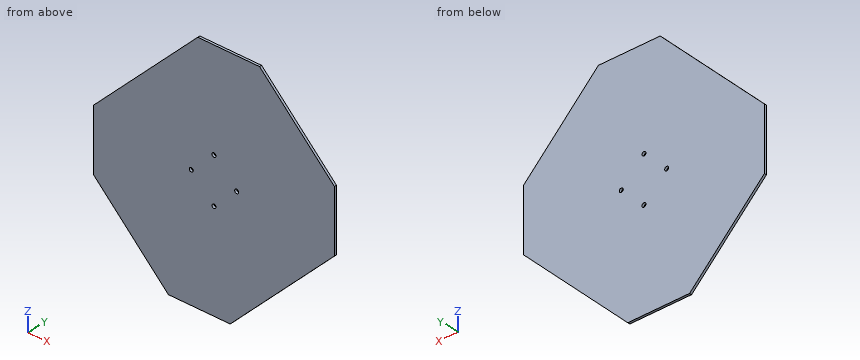
```python
from build123d import *

# Parameters (mm, degrees)
BOSS_EXTRUDE2_DEPTH              = 3
F_13_64_0_20313_DIAMETER_HOLE1_D = 5.159502


with BuildPart() as part:
    # Sketch3 → Boss-Extrude2 (new body)
    with BuildSketch(Plane(origin=(0, 0, 0), x_dir=(1, 0, 0), z_dir=(0, 1, 0))):
        Polygon((146.917568262, 30.566233816), (11.506619665, 165.977182413), (-68.75, 165.977182413), (-165.977182413, 68.75), (-165.977182413, -11.506619665), (-30.566233816, -146.917568262), (49.690385849, -146.917568262), (146.917568262, -49.690385849), align=None)
    extrude(amount=BOSS_EXTRUDE2_DEPTH)

    # 13/64 (0.20313) Diameter Hole1 (through all)
    with Locations(Plane(origin=(0, 0, 0), x_dir=(-1, 0, 0), z_dir=(0, -1, 0))):
        with Locations((39.029807033, 9.528212544), (9.528212544, -19.970192881), (-19.970192881, 9.531401607), (9.531401607, 39.029807033)):
            Hole(F_13_64_0_20313_DIAMETER_HOLE1_D / 2)


solid = part.part
```
Could you check a few things on this model? Use its own coordinates, in mm. Give positions to 0.01 mm unless a question says otherwise; leave off trailing zeros. Order: outer loops, then holes, each group sorted by start corner. A loop starts at its lowest first (then second) coordinate and runs counter-clockwise, first axis right, second up.
Q1. Suppose I cut it at B-B, the plane z = -89. Write out the boundary of the cut face in (x, y).
Q2. Suppose I cut it at C-C, the plane x = -76. Write out the boundary of the cut face in (y, z), and give its area (3 significant figures).
Q3. I'm going to push a flat-ended pin straight in: P1, Ø8.5, axis at x = -9.53, z = -39.03, coming from the +Y side. Where does the tip first touch, or does it pass through?
Q4. If I drill on line 1 along X through (y, z) = (2.75, 21); line 2 along X through (y, z) = (1.55, 19.5); line 3 along Z through (x, y) = (-38.5, 0.8), over which ranges is the centre line in solid material (lowest first)?
Q5. Suppose I cut it at A-A, the plane y = 0.8. Write out the boundary of the cut face in (x, z), and give its area (3 significant figures).
Solution:
1. outline: (-145.73, 0) - (88.48, 0) - (88.48, 3) - (-145.73, 3) - close
2. outline: (0, -158.73) - (3, -158.73) - (3, 101.48) - (0, 101.48) - close
2. area: 781 mm2
3. P1: stops at y = 3
4. line 1: x = -156.48 to -11.89, -7.16 to 146.92
4. line 2: x = -157.98 to -12.06, -6.99 to 146.92
4. line 3: z = -165.98 to -12.05, -7 to 138.98
5. outline: (-165.98, -68.75) - (-68.75, -165.98) - (11.51, -165.98) - (146.92, -30.57) - (146.92, 49.69) - (49.69, 146.92) - (-30.57, 146.92) - (-165.98, 11.51) - close; hole circle Ø5.16 at (-39.03, -9.53); hole circle Ø5.16 at (-9.53, -39.03); hole circle Ø5.16 at (-9.53, 19.97); hole circle Ø5.16 at (19.97, -9.53)
5. area: 70,000 mm2
